The listing builds one solid part. Answer for the finished solid, in the listing's coordinates (mm). Face numbers are marked on the shaded views. A direction names the side the tool comes from. Round coordinates to 2 decimals unless told otherwise and drop trailing zeros. Write each loop counter-clockwise with the first axis right and the second up, starting at its lowest first coordinate (ties: lowest second). Pieces come first, ordered by that corner, then holes. Notation, with made-up numbers: (33.5, -19) - (70.5, -19) arc R16 cw to (70.5, 7) - close; hole circle Ø10 at (29.5, 29.5). An arc over 180 degrees is marked (long way). Return JSON: item names as keys, results as strings. Group by question number.
from build123d import *

# Parameters (mm, degrees)
SKETCH1_W                       = 22
SKETCH1_H                       = 23
BOSS_EXTRUDE1_DEPTH             = 32
FILLET1_R                       = 3
CBORE_FOR_M2_SHCS1_D            = 2.4
CBORE_FOR_M2_SHCS1_CBORE_D      = 4.4
CBORE_FOR_M2_SHCS1_CBORE_DEPTH  = 21
F_5_0MM_DOWEL_HOLE1_D           = 5.2
F_5_0MM_DOWEL_HOLE1_DEPTH       = 4
F_5_0MM_DOWEL_HOLE1_CSINK_D     = 5.4
F_5_0MM_DOWEL_HOLE1_CSINK_ANGLE = 70
FILLET2_R                       = 2
M3_CLEARANCE_HOLE1_D            = 3.4
M3_CLEARANCE_HOLE1_DEPTH        = 7.5
M3_CLEARANCE_HOLE1_TIP          = 1.021463052


with BuildPart() as part:
    # Sketch1 → Boss-Extrude1 (new body)
    with BuildSketch(Plane(origin=(0, 0, 0), x_dir=(1, 0, 0), z_dir=(0, 1, 0))):
        with Locations((11, 11.5)):
            Rectangle(SKETCH1_W, SKETCH1_H)
        Polygon((4, 4), (18, 4), (18, 9), (11, 16), (4, 9), align=None, mode=Mode.SUBTRACT)
    extrude(amount=BOSS_EXTRUDE1_DEPTH)

    # Fillet1
    fillet1_edges = [part.edges().sort_by_distance(p)[0] for p in [
        (4, 16, -9),
        (4, 16, -4),
        (18, 16, -4),
        (18, 16, -9),
    ]]
    fillet(fillet1_edges, radius=FILLET1_R)

    # CBORE for M2 SHCS1 (through all)
    with Locations(Plane.XY):
        with Locations((5, 12), (17, 12), (17, 20), (5, 20)):
            CounterBoreHole(CBORE_FOR_M2_SHCS1_D / 2, CBORE_FOR_M2_SHCS1_CBORE_D / 2, CBORE_FOR_M2_SHCS1_CBORE_DEPTH)

    # Ø5.0mm Dowel Hole1
    with Locations(Plane.XY):
        with Locations((11, 16)):
            CounterSinkHole(F_5_0MM_DOWEL_HOLE1_D / 2, F_5_0MM_DOWEL_HOLE1_CSINK_D / 2, depth=F_5_0MM_DOWEL_HOLE1_DEPTH, counter_sink_angle=F_5_0MM_DOWEL_HOLE1_CSINK_ANGLE)

    # Fillet2
    fillet2_edges = [part.edges().sort_by_distance(p)[0] for p in [
        (0, 16, 0),
        (0, 16, -23),
        (22, 16, -23),
        (22, 16, 0),
    ]]
    fillet(fillet2_edges, radius=FILLET2_R)

    # M3 Clearance Hole1
    with Locations(Plane(origin=(0, 32, 0), x_dir=(1, 0, 0), z_dir=(0, 1, 0))):
        with Locations((4, 20), (19, 20)):
            Hole(M3_CLEARANCE_HOLE1_D / 2, depth=M3_CLEARANCE_HOLE1_DEPTH)
            with Locations((0, 0, -(M3_CLEARANCE_HOLE1_DEPTH + M3_CLEARANCE_HOLE1_TIP / 2))):  # 118° drill point
                Cone(0, M3_CLEARANCE_HOLE1_D / 2, M3_CLEARANCE_HOLE1_TIP, mode=Mode.SUBTRACT)


solid = part.part
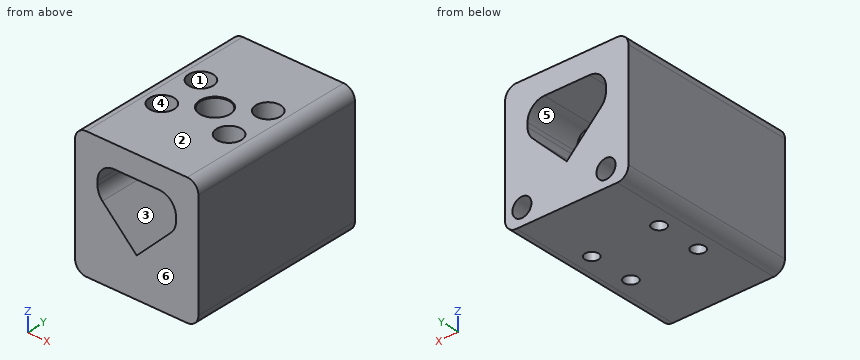
(1) For the marked faces 4, 5 and 6, determine the directions among +Z, -Z, +X, -X, +Y, -Y from which every point of the face is accessible in a straight line to the end or side of a thin tool.
(2) Consider line 1 (Y direction, x = 17, z = -22.5); line 2 (Y direction, x = 5, z = -15.5); line 3 (Z direction, x = 19, y = 28.75). Determine where each line is inside the solid, lowest interval first.
(3) Determine the mould class of the marked faces 1, 2 and 3 for opening direction Z: +Z half, -Z half, draft (parallel to the pull), parting line (faces both ways), or undercut.
(4) Find section D-D (z = -5.5). Write down the section's boundary in (x, y), plus the area to 3 significant figures.
(5) Find section C-C (y = 3.5). Write down the section's boundary in (x, z), plus the area to 3 significant figures.
(6) Find section A-A (y = 20). State how many separate pieces and enclosed holes the cut face has, plus the area to 3 significant figures.
(7) Find section B-B (y = 28). Write down the section's boundary in (x, z), plus the area to 3 significant figures.
(8) Flat-ended cylindrical pins translate along their axes: pin 1 (5 mm diameter, centred on x = 3.5, y = 18, fed in from +Z); pin 2 (1.3 mm diameter, centred on x = 4.5, y = 12, fed in from +Z); pin 3 (4 mm diameter, centred on x = 5, y = 20, fed in from +Z). Find the tip coordinate at first contact, or state that the pin passes through.
Check sheet entries:
{
 "1": {"face 4": "+Z", "face 5": "+Y, -Y", "face 6": "+Z, -Z, +X, -X, -Y"},
 "2": {"line 1": "y = 0 to 10.8, 13.2 to 18.8, 21.2 to 32", "line 2": "y = 0 to 9.8, 14.2 to 17.8, 22.2 to 32", "line 3": "z = -23 to -21.7, -18.3 to 0"},
 "3": {"face 1": "draft", "face 2": "+Z half", "face 3": "undercut"},
 "4": {"outline": "(0, 0) - (4.4, 0) - (4.4, 9.88) arc R2.2 cw to (4.4, 14.12) - (4.4, 17.88) arc R2.2 cw to (4.4, 22.12) - (4.4, 32) - (0, 32) - close; (17.6, 0) - (22, 0) - (22, 32) - (17.6, 32) - (17.6, 22.12) arc R2.2 cw to (17.6, 17.88) - (17.6, 14.12) arc R2.2 cw to (17.6, 9.88) - close", "area": "262 mm^2"},
 "5": {"outline": "(0, -21) arc R2 ccw to (2, -23) - (20, -23) arc R2 ccw to (22, -21) - (22, -2) arc R2 ccw to (20, 0) - (2, 0) arc R2 ccw to (0, -2) - close; hole (4, -7.76) arc R3 ccw to (4.88, -9.88) - (11, -16) - (17.12, -9.88) arc R3 ccw to (18, -7.76) - (18, -7) arc R3 ccw to (15, -4) - (7, -4) arc R3 ccw to (4, -7) - close", "area": "388 mm^2"},
 "6": {"separate pieces": "4", "enclosed holes": "0", "area": "231 mm^2"},
 "7": {"outline": "(0, -21) arc R2 ccw to (2, -23) - (20, -23) arc R2 ccw to (22, -21) - (22, -2) arc R2 ccw to (20, 0) - (2, 0) arc R2 ccw to (0, -2) - close; hole circle Ø3.4 at (4, -20); hole (4, -7.76) arc R3 ccw to (4.88, -9.88) - (11, -16) - (17.12, -9.88) arc R3 ccw to (18, -7.76) - (18, -7) arc R3 ccw to (15, -4) - (7, -4) arc R3 ccw to (4, -7) - close; hole circle Ø3.4 at (19, -20)", "area": "370 mm^2"},
 "8": {"pin 1": "stops at z = 0", "pin 2": "passes through", "pin 3": "stops at z = -21"}
}
